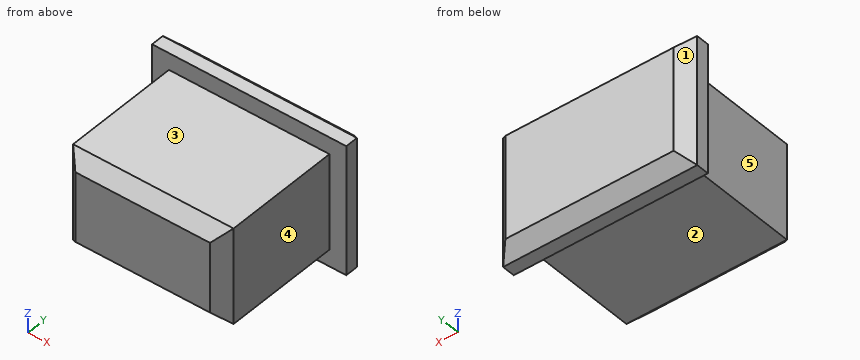
```python
from build123d import *

# Parameters (mm, degrees)
SKETCH_1_W      = 15
SKETCH_1_H      = 10
SKETCH_1_W_2    = 12.4
SKETCH_1_H_2    = 7.4
EXTRUDE_1_DEPTH = 2
SKETCH_2_W      = 12.4
SKETCH_2_H      = 7.4
EXTRUDE_2_DEPTH = 10
CHAMFER_1_SIZE  = 1
CHAMFER_2_SIZE  = 1


with BuildPart() as part:
    # ｽｹｯﾁ1 → ﾎﾞｽ - 押し出し1 (new body)
    # profile 1 of 2: a face of its own
    with BuildSketch(Plane(origin=(0, 0, 0), x_dir=(1, 0, 0), z_dir=(0, 1, 0))):
        Rectangle(SKETCH_1_W, SKETCH_1_H)
        Rectangle(SKETCH_1_W_2, SKETCH_1_H_2, mode=Mode.SUBTRACT)
    # profile 2 of 2: a face of its own
    with BuildSketch(Plane(origin=(0, 0, 0), x_dir=(1, 0, 0), z_dir=(0, 1, 0))):
        Rectangle(SKETCH_1_W_2, SKETCH_1_H_2)
    extrude(amount=EXTRUDE_1_DEPTH)

    # ｽｹｯﾁ2 → ﾎﾞｽ - 押し出し2 (add)
    with BuildSketch(Plane.XZ):
        Rectangle(SKETCH_2_W, SKETCH_2_H)
    extrude(amount=EXTRUDE_2_DEPTH)

    # 面取り1
    chamfer_1_edges = [part.edges().sort_by_distance(p)[0] for p in [
        (0, -10, 3.7),
        (-6.2, -10, 0),
        (0, -10, -3.7),
        (6.2, -10, 0),
    ]]
    chamfer(chamfer_1_edges, length=CHAMFER_1_SIZE)

    # 面取り2
    chamfer_2_edges = [part.edges().sort_by_distance(p)[0] for p in [
        (0, 2, -5),
        (-7.5, 2, 0),
        (0, 2, 5),
        (7.5, 2, 0),
    ]]
    chamfer(chamfer_2_edges, length=CHAMFER_2_SIZE)


solid = part.part
```
Verification items for the finished model (mm, model axes). Face numbers are marked on the shaded views. A direction names the side the tool comes from. Coordinates: 2 decimals unless noted, no trailing zeros. Loops run counter-clockwise (first coordinate to the right, second up) from the corner with the lowest first, then second, coordinate; pieces in that order, holes last. Notation, with made-up numbers: (-28.75, 70) - (-1.75, 70) arc R8 ccw to (-1.75, 75) - close; hole circle Ø9 at (27.5, 43.25). An arc over 180 degrees is marked (long way). Answer as a JSON object with one key per item and string values.
(1) Access from +Z, -Z, +X, -X, +Y, -Y to the whole of each face (thin tool, end or side, straight path). Record for the marked faces 1, 2, 3, 4 and 5.
Response:
{"face 1": "+Z, -Z, -X, +Y", "face 2": "-Z, +X, -X, -Y", "face 3": "+Z, +X, -X, -Y", "face 4": "+Z, -Z, +X, -Y", "face 5": "+Z, -Z, -X, -Y"}
(2) Cross-section at A-A, the plane z = 3.5. Record the boundary of the cut face in (x, y).
Response:
{"outline": "(-7.5, 0) - (-6.2, 0) - (-6.2, -9) - (-6, -9.2) - (6, -9.2) - (6.2, -9) - (6.2, 0) - (7.5, 0) - (7.5, 1) - (6.5, 2) - (-6.5, 2) - (-7.5, 1) - close"}
(3) Cross-section at C-C, the plane y = -0.5. Record the boundary of the cut face in (x, z), then the cut area to 3 significant figures.
Response:
{"outline": "(-6.2, -3.7) - (6.2, -3.7) - (6.2, 3.7) - (-6.2, 3.7) - close", "area": "91.8 mm²"}
(4) Go/stop test with flat-tipped pins: pin 1 Ø1 at (x, y) = (1, -8.5) entering from +Z; pin 2 Ø6 at (y, z) = (-4.5, -1) entering from -X; pin 3 Ø2.5 at (x, y) = (-1.5, -3.5) entering from -Z. Record where each tip stops, or that it passes through.
Response:
{"pin 1": "stops at z = 3.7", "pin 2": "stops at x = -6.2", "pin 3": "stops at z = -3.7"}
(5) Cross-section at B-B, the plane x = 0.5. Record the boundary of the cut face in (y, z), then the cut area to 3 significant figures.
Response:
{"outline": "(-10, -2.7) - (-9, -3.7) - (0, -3.7) - (0, -5) - (1, -5) - (2, -4) - (2, 4) - (1, 5) - (0, 5) - (0, 3.7) - (-9, 3.7) - (-10, 2.7) - close", "area": "92.0 mm²"}
(6) Scan lines: line 1 along Z through (x, y) = (-4.25, -0.25); line 2 along X through (y, z) = (-6, 0.25); line 3 along Y through (x, z) = (6.25, 0.75). Record each from-to range of solid material in increasing order.
Response:
{"line 1": "z = -3.7 to 3.7", "line 2": "x = -6.2 to 6.2", "line 3": "y = 0 to 2"}
